from build123d import *

# Parameters (mm, degrees)
BOSS_EXTRUDE1_DEPTH                           = 3
CSK_FOR_5_FLAT_HEAD_SOCKET_CAP_SCREW1_A_COUNT = 2
CSK_FOR_5_FLAT_HEAD_SOCKET_CAP_SCREW1_A_PITCH = 56.41402705
CSK_FOR_5_FLAT_HEAD_SOCKET_CAP_SCRE_2_COUNT   = 2
CSK_FOR_5_FLAT_HEAD_SOCKET_CAP_SCRE_2_PITCH   = 80.02134109
CSK_FOR_5_FLAT_HEAD_SOCKET_CAP_SCRE_3_COUNT   = 2
CSK_FOR_5_FLAT_HEAD_SOCKET_CAP_SCRE_3_PITCH   = 46.660638534


with BuildPart() as part:
    # Sketch1 → Boss-Extrude1 (new body)
    with BuildSketch(Plane.XY):
        Polygon((-25.209392257, 17.065862145), (-32.589765844, 17.616547994), (-33.185013977, 9.638724086), (-25.804640414, 9.088037903), (-28.980934475, -33.481127138), (-11.529359642, -34.783274677), (-12.124624122, -42.761097701), (-4.146801098, -43.356362181), (-3.551536618, -35.378539157), (-2.025288651, -14.922973048), (34.074511236, -17.616481792), (34.672848055, -17.661125404), (35.268112443, -9.683303605), (26.697352489, -9.043797194), (29.87364655, 33.525367847), (13.014992274, 34.783274677), (13.610256754, 42.761097701), (5.63243373, 43.356362181), (5.03716925, 35.378539157), (3.51996828, 15.044798681), align=None)
    extrude(amount=BOSS_EXTRUDE1_DEPTH)

    # Sketch2 → CSK for #5 Flat Head Socket Cap Screw1 (revolve, cut)
    with BuildSketch(Plane(origin=(-7.973395272, -39.059721921, 3), x_dir=(0, -1, 0), z_dir=(1, 0, 0))):
        Polygon((0, 0), (0, 3), (1.7272, 3), (1.7272, 2.118403422), (3.5687, 0), align=None)
    csk_for_5_flat_head_socket_cap_screw1 = revolve(axis=Axis((-7.973395272, -39.059721921, 9.35), (0, 0, -1)), mode=Mode.SUBTRACT)

    # CSK for #5 Flat Head Socket Cap Screw1 a: CSK for #5 Flat Head Socket Cap Screw1 ×2
    with Locations(*[Vector(-0.370919862, 0.928664878, 0) * (i * CSK_FOR_5_FLAT_HEAD_SOCKET_CAP_SCREW1_A_PITCH) for i in range(1, CSK_FOR_5_FLAT_HEAD_SOCKET_CAP_SCREW1_A_COUNT)]):
        add(csk_for_5_flat_head_socket_cap_screw1, mode=Mode.SUBTRACT)

    # CSK for _5 Flat Head Socket Cap Scre 2: CSK for #5 Flat Head Socket Cap Screw1 ×2
    with Locations(*[Vector(0.216156191, 0.976358797, 0) * (i * CSK_FOR_5_FLAT_HEAD_SOCKET_CAP_SCRE_2_PITCH) for i in range(1, CSK_FOR_5_FLAT_HEAD_SOCKET_CAP_SCRE_2_COUNT)]):
        add(csk_for_5_flat_head_socket_cap_screw1, mode=Mode.SUBTRACT)

    # CSK for _5 Flat Head Socket Cap Scre 3: CSK for #5 Flat Head Socket Cap Screw1 ×2
    with Locations(*[Vector(0.834857059, 0.550466794, 0) * (i * CSK_FOR_5_FLAT_HEAD_SOCKET_CAP_SCRE_3_PITCH) for i in range(1, CSK_FOR_5_FLAT_HEAD_SOCKET_CAP_SCRE_3_COUNT)]):
        add(csk_for_5_flat_head_socket_cap_screw1, mode=Mode.SUBTRACT)


solid = part.part
Design review of the part built by this model. Coordinates are the model's own, in mm. A direction names the side the tool comes from. Round coordinates to 2 decimals unless told otherwise and drop trailing zeros. Loops run counter-clockwise (first coordinate to the right, second up) from the corner with the lowest first, then second, coordinate; pieces in that order, holes last. Notation, with made-up numbers: (-11, 85) -> (-4, 85) arc R11 cw to (-4, 101) -> close; hole circle Ø9 at (-27, 81). An arc over 180 degrees is marked (long way). Use one line per item in the form item = value. Start each with the question number.
Q1. Draft analysis for pull direction X (two halves, no side actions). For faces 1 (the face through (32.103, -11.913, 1.014)), 2 (the face through (-11.823, -38.716, 1.479)), 3 (the face through (9.677, 43.055, 1.479)), state which applies: +X half, -X half, draft (parallel to the pull), parting line (faces both ways), or undercut.
Q2. For pin 1 Ø3 at (x, y) = (-15.5, 14) entering from -Z; pin 2 Ø1.5 at (y, z) = (17.5, 2.5) entering from +X; pin 3 Ø4 at (x, y) = (-28.9, 13.33) entering from +Z, all flat-tipped, find the tip position at first contact; note any pin that passes through.
Q3. We need section C-C on y = -24. Give the boundary of the cut face in (x, z).
Q4. Machinability: for faces 4 (the face through (34.966, -13.728, 1.479)), 5 (the face through (-10.64, 16.04, 1.48)), 6 (the face through (31.043, -9.368, 1.479)), which of the approach directions +Z, -Z, +X, -X, +Y, -Y give a long, thin tool a straight path to every point of the face, cutting with its end or side? Answer none if there is none.
Q5. Wall thickness on line 1 along Y through (x, z) = (31.5, 1.9); line 2 along Y through (x, z) = (9, 0.5); line 3 along X through (y, z) = (18.5, 1.6): over which ranges is each line inside the solid? List them lowest first. Write a range as [from, to].
Q6. We need section B-B on x = 0.5. Give the boundary of the cut face in (y, z), then the cut area to 3 significant figures.
Q7. We need section A-A on z = 2.3. Give the boundary of the cut face in (x, y) (3 decimals), then the cut area to 3 significant figures.
Calculated:
q1.face_1 = undercut
q1.face_2 = -X half
q1.face_3 = +X half
q2.pin_1 = 0
q2.pin_2 = 28.73
q2.pin_3 = 1.2
q3.outline = (-28.27, 0) -> (-2.7, 0) -> (-2.7, 3) -> (-28.27, 3) -> close
q4.face_4 = +Z, -Z, +X, -Y
q4.face_5 = +Z, -Z, +Y
q4.face_6 = +Z, -Z, +X
q5.line_1 = [-17.42, -15.94], [-10.81, -9.4]
q5.line_2 = [-15.75, 37.37], [40.77, 43.11]
q5.line_3 = [3.78, 28.75]
q6.outline = (-15.11, 0) -> (15.26, 0) -> (15.26, 3) -> (-15.11, 3) -> close
q6.area = 91.1 mm²
q7.outline = (-33.185, 9.639) -> (-25.805, 9.088) -> (-28.981, -33.481) -> (-11.529, -34.783) -> (-12.125, -42.761) -> (-4.147, -43.356) -> (-3.552, -35.379) -> (-2.025, -14.923) -> (34.673, -17.661) -> (35.268, -9.683) -> (26.697, -9.044) -> (29.874, 33.525) -> (13.015, 34.783) -> (13.61, 42.761) -> (5.632, 43.356) -> (3.52, 15.045) -> (-25.209, 17.066) -> (-32.59, 17.617) -> close; hole circle Ø5.92 at (-28.898, 13.33); hole circle Ø5.92 at (-7.973, -39.06); hole circle Ø5.92 at (9.324, 39.07); hole circle Ø5.92 at (30.982, -13.375)
q7.area = 2,800 mm²
